from build123d import *

# Parameters (mm, degrees)
BODY_DEPTH          = 21
SKETCH2_R           = 0.85
BOLT_HOLE_DEPTH     = 22
SKETCH3_W           = 6
SKETCH3_H           = 6.5
BOSS_EXTRUDE1_DEPTH = 20
SKETCH4_R           = 1.6
CUT_EXTRUDE1_DEPTH  = 24
EDGE_FILLETS_R      = 1


with BuildPart() as part:
    # Sketch1 → body (new body)
    with BuildSketch(Plane(origin=(0, 0, 0), x_dir=(0, 0, -1), z_dir=(1, 0, 0))):
        Polygon((0, 0), (10, 0), (0, -10), align=None)
    extrude(amount=BODY_DEPTH)

    # Sketch2 → bolt_hole (cut, through all)
    with BuildSketch(Plane.ZY):
        with Locations((-3, -3)):
            Circle(SKETCH2_R)
    extrude(amount=-BOLT_HOLE_DEPTH, mode=Mode.SUBTRACT)

    # Sketch3 → Boss-Extrude1 (add)
    with BuildSketch(Plane.XY):
        with Locations((2, 3.25)):
            Rectangle(SKETCH3_W, SKETCH3_H)
        with Locations((19, 3.25)):
            Rectangle(SKETCH3_W, SKETCH3_H)
    extrude(amount=-BOSS_EXTRUDE1_DEPTH)

    # Sketch4 → Cut-Extrude1 (cut, through all)
    with BuildSketch(Plane(origin=(22, 0, 0), x_dir=(0, 0, -1), z_dir=(1, 0, 0))):
        with Locations((16.8, 3.25)):
            Circle(SKETCH4_R)
    extrude(amount=-CUT_EXTRUDE1_DEPTH, mode=Mode.SUBTRACT)

    # edge_fillets
    edge_fillets_edges = [part.edges().sort_by_distance(p)[0] for p in [
        (21, -5, 0),
        (21, -5, -5),
        (2, 0, -20),
        (-1, 3.25, -20),
        (2, 6.5, -20),
        (-1, 6.5, -10),
        (5, 3.25, -20),
        (5, 6.5, -10),
        (-0.5, 0, 0),
        (5, 3.25, 0),
        (2, 6.5, 0),
        (10.5, 0, 0),
        (22, 3.25, -20),
        (22, 6.5, -10),
        (19, 0, -20),
        (16, 3.25, -20),
        (19, 6.5, -20),
        (16, 6.5, -10),
        (19, 6.5, 0),
        (21.5, 0, 0),
        (0, -5, -5),
        (0, -5, 0),
        (10.5, -10, 0),
    ]]
    fillet(edge_fillets_edges, radius=EDGE_FILLETS_R)


solid = part.part
Can you work these out from the model? Positions are in its coordinate system, mm. A direction names the side the tool comes from. Round coordinates to 2 decimals unless told otherwise and drop trailing zeros. Loops run counter-clockwise (first coordinate to the right, second up) from the corner with the lowest first, then second, coordinate; pieces in that order, holes last. Notation, with made-up numbers: (45.5, 65.5) - (99.5, 65.5) arc R25 cw to (99.5, 98.5) - close; hole circle Ø3 at (44.25, 33). An arc over 180 degrees is marked (long way). Use CSV: the item, a comma, the result in double quotes. Start each with the question number.
1) If we section it at B-B on x = 2: Write out the boundary of the cut face in (y, z).
2) For faces 1 (the cylindrical face through (-0.2, 0.4, -0.2)), 2 (the flat face through (21, -2, -4)), 3 (the cylindrical face through (21.2, 0.4, -0.2)), 4 (the flat face through (20, 0, -14)), which set-ups out of +Z, -Z, +X, -X, +Y, -Y let a thin tool reach every point of the face, with its end or its side?
3) If we section it at A-A on y = 3.25: Write out the boundary of the cut face in (x, z), plus the area to 3 significant figures.
4) If we section it at D-D on z = -16.8: Write out the boundary of the cut face in (x, y).
5) Please list where these lines run through material, in increasing order: probe 1 along X at (y, z) = (2, -2); probe 2 along Y at (x, z) = (14.75, -3); probe 3 along Y at (x, z) = (1.6, -16.8). Write a range as [from, to].
6) If we section it at C-C on z = -10.5: Write out the boundary of the cut face in (x, y), plus the area to 3 significant figures.
7) We'd pull the mould along X, two halves only. Please class faces 5 (the cylindrical face through (16.285, 2.788, -19.699)), 6 (the cylindrical face through (2.028, 6.199, -19.715)), 7 (the cylindrical face through (0.301, -3.233, -0.285)), 8 (the flat face through (10, 0, -5)): released by +X, released by -X, zero draft, split by the parting line, or undercut.
8) For pin 1 Ø8.5 at (y, z) = (-5.5, -6) entering from +X; pin 2 Ø1 at (x, z) = (17, -15.5) entering from -Y; pin 3 Ø2.5 at (y, z) = (-4.5, -6.5) entering from -X, each with a flat end and sliding along its axis, tell me the tip position at first contact or that it passes through.
Geometry results:
1,outline,"(-8.29, -1.71) - (0, -10) - (0, -19) arc R1 ccw to (1, -20) - (5.5, -20) arc R1 ccw to (6.5, -19) - (6.5, -1) arc R1 ccw to (5.5, 0) - (-7.59, 0) arc R1 ccw to start; hole circle Ø1.7 at (-3, -3); hole circle Ø3.2 at (3.25, -16.8)"
2,face 1,"+Z, -X, -Y"
2,face 2,"+Z, -Z, +X, -Y"
2,face 3,"+Z, +X, -Y"
2,face 4,"-Z, +X, -Y"
3,outline,"(-1, -19) arc R1 ccw to (0, -20) - (4, -20) arc R1 ccw to (5, -19) - (5, -18.4) - (-1, -18.4) - close; (-1, -15.2) - (5, -15.2) - (5, -1) arc R1 ccw to (4, 0) - (-1, 0) - close; (16, -19) arc R1 ccw to (17, -20) - (21, -20) arc R1 ccw to (22, -19) - (22, -18.4) - (16, -18.4) - close; (16, -15.2) - (22, -15.2) - (22, 0) - (16, 0) - close"
3,area,"201 mm2"
4,outline,"(-1, 0) - (5, 0) - (5, 1.65) - (-1, 1.65) - close; (-1, 4.85) - (5, 4.85) - (5, 5.5) arc R1 ccw to (4, 6.5) - (0, 6.5) arc R1 ccw to (-1, 5.5) - close; (16, 0) - (22, 0) - (22, 1.65) - (16, 1.65) - close; (16, 4.85) - (22, 4.85) - (22, 5.5) arc R1 ccw to (21, 6.5) - (17, 6.5) arc R1 ccw to (16, 5.5) - close"
5,probe 1,"x = [-1, 5], [16, 22]"
5,probe 2,"y = [-7, -3.85], [-2.15, 0]"
5,probe 3,"y = [0, 1.65], [4.85, 6.5]"
6,outline,"(-1, 0) - (5, 0) - (5, 5.5) arc R1 ccw to (4, 6.5) - (0, 6.5) arc R1 ccw to (-1, 5.5) - close; (16, 0) - (22, 0) - (22, 5.5) arc R1 ccw to (21, 6.5) - (17, 6.5) arc R1 ccw to (16, 5.5) - close"
6,area,"77.1 mm2"
7,face 5,"undercut"
7,face 6,"zero draft"
7,face 7,"released by -X"
7,face 8,"undercut"
8,pin 1,"stops at x = 21"
8,pin 2,"stops at y = 0"
8,pin 3,"stops at x = 0.11"
